from build123d import *

# Parameters (mm, degrees)
F1_DEPTH = 150


with BuildPart() as f1:
    # F0 (on Right) → F1 (new body)
    with BuildSketch(Plane.YZ):
        with BuildLine():
            Line((-125, 0), (0, 0))
            Line((0, 0), (125, 0))
            ThreePointArc((125, 0), (128.535534, 1.464466), (130, 5))
            Line((130, 5), (130, 175))
            ThreePointArc((130, 175), (128.535534, 178.535534), (125, 180))
            Line((125, 180), (105, 180))
            ThreePointArc((105, 180), (101.464466, 178.535534), (100, 175))
            Line((100, 175), (100, 35))
            ThreePointArc((100, 35), (98.535534, 31.464466), (95, 30))
            Line((95, 30), (0, 30))
            Line((0, 30), (-95, 30))
            ThreePointArc((-95, 30), (-98.535534, 31.464466), (-100, 35))
            Line((-100, 35), (-100, 175))
            ThreePointArc((-100, 175), (-101.464466, 178.535534), (-105, 180))
            Line((-105, 180), (-125, 180))
            ThreePointArc((-125, 180), (-128.535534, 178.535534), (-130, 175))
            Line((-130, 175), (-130, 5))
            ThreePointArc((-130, 5), (-128.535534, 1.464466), (-125, 0))
        make_face()
    extrude(amount=F1_DEPTH)


solid = f1.part
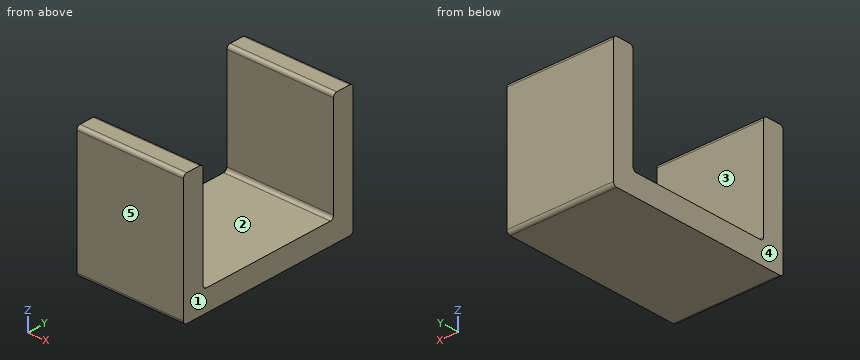
Verification items for the finished model (mm, model axes). Face numbers are marked on the shaded views. A direction names the side the tool comes from. Give positions to 0.01 mm unless a question says otherwise; leave off trailing zeros. Order: outer loops, then holes, each group sorted by start corner. A loop starts at its lowest first (then second) coordinate and runs counter-clockwise, first axis right, second up. Notation, with made-up numbers: M 10,85.5 L 26,85.5 A30 ccw 26,108.5 Z; hole C 77,15.5 d5. An arc over 180 degrees is marked long. Answer as a JSON object with one key per item and string values. Group by question number.
1) Cross-section at B-B (x = 41). Enter the section's corners in (y, z), then the cut area to 3 significant figures.
2) Access from +Z, -Z, +X, -X, +Y, -Y to the whole of each face (thin tool, end or side, straight path). Record for the marked faces 1 and 2.
3) Scan lines: line 1 along Y through (x, z) = (45, 62); line 2 along Z through (x, y) = (135, 75). Record each from-to range of solid material in increasing order. Write a range as [from, to].
4) Cross-section at A-A (z = 161.5). Enter the section's corners in (x, y).
5) Depth check by flat-ended pin: pin 1 Ø4 at (y, z) = (70, 25) entering from -X; pin 2 Ø4 at (x, y) = (120.5, -17) entering from +Z. Enter the tip coordinate at first touch or a pass-through.
6) Mould release check, pull along Y, two halves, no side actions. Record for the marked faces 3, 4 and 5: released by +Y, released by -Y, zero draft, split by the parting line, or undercut.
7) Cross-section at C-C (y = 75.5). Enter the section's corners in (x, z).
Result sheet:
{
 "1": {"outline": "M -130,5 A5 ccw -125,0 L 125,0 A5 ccw 130,5 L 130,175 A5 ccw 125,180 L 105,180 A5 ccw 100,175 L 100,35 A5 cw 95,30 L -95,30 A5 cw -100,35 L -100,175 A5 ccw -105,180 L -125,180 A5 ccw -130,175 Z", "area": "16,800 mm2"},
 "2": {"face 1": "+Z, -Z, +X, +Y, -Y", "face 2": "+Z, +X, -X"},
 "3": {"line 1": "y = [-130, -100], [100, 130]", "line 2": "z = [0, 30]"},
 "4": {"outline": "M 0,-130 L 150,-130 L 150,-100 L 0,-100 Z; M 0,100 L 150,100 L 150,130 L 0,130 Z"},
 "5": {"pin 1": "stops at x = 0", "pin 2": "stops at z = 30"},
 "6": {"face 3": "undercut", "face 4": "zero draft", "face 5": "released by -Y"},
 "7": {"outline": "M 0,0 L 150,0 L 150,30 L 0,30 Z"}
}
